Source: CAD feature listing. Evaluate the final solid. Frame: model axes, mm. A direction names the side the tool comes from. Round coordinates to 2 decimals unless told otherwise and drop trailing zeros.
```python
from build123d import *


with BuildPart() as part:
    # Sketch2 → Revolve2 (revolve)
    with BuildSketch(Plane(origin=(0, 0, 0), x_dir=(0, 0, -1), z_dir=(1, 0, 0)), mode=Mode.PRIVATE) as revolve2_sk:
        with BuildLine():
            Line((0, 0), (31, 0))
            Line((31, 0), (31, 9))
            Line((31, 9), (24.583151623, 9))
            ThreePointArc((24.583151623, 9), (19.839895343, 11.325558565), (18.773545819, 16.499493381))
            Line((18.773545819, 16.499493381), (22, 29))
            Line((22, 29), (22, 35))
            Line((22, 35), (18, 35))
            Line((18, 35), (13.354094276, 17))
            Line((13.354094276, 17), (8.876757203, 17))
            Line((8.876757203, 17), (4, 34.552318614))
            Line((4, 34.552318614), (0, 34.552318614))
            Line((0, 34.552318614), (0, 28.552318614))
            Line((0, 28.552318614), (4.37578125, 12.803101771))
            ThreePointArc((4.37578125, 12.803101771), (3.873716269, 10.184690841), (1.485274798, 9))
            Line((1.485274798, 9), (0, 9))
            Line((0, 9), (0, 0))
        make_face()
    revolve(revolve2_sk.sketch.rotate(Axis((0, -15, 0), (0, 0, -1)), 90), axis=Axis((0, -15, 0), (0, 0, -1)))


solid = part.part
```
Q1. Line query: line 1 (Y direction, x = 0, z = -10); line 2 (Y direction, x = 0, z = -18.5); line 3 (Z direction, x = -46, y = -22). Output: solid intervals per line, ascending.
Q2. Set-up query: faces 1 (the face through (22.89, -22.21, -27.75)), 2 (the face through (47.264, -29.884, -1.972)), 3 (the face through (-4.28, -47.59, -13.58)). Return all of +Z, -Z, +X, -X, +Y, -Y with unobstructed straight access to the full face (end or side cutting, diameter ignored); none if empty.
Q3. Pin query (flat end, axial travel): P1, Ø2, axis at x = -21, z = -12, coming from the +Y side; P2, Ø1, axis at x = -29, y = -10, coming from the -Z side; P3, Ø3, axis at y = 2.5, z = -21, coming from the +X side. Return the tip coordinate at first contact, or that it passes through.
Q4. Mould query, pull axis Z, two halves, no side actions, for faces 4 (the face through (-6.94, 16.24, -11.08)), 5 (the face through (0.2, 29.2, -22)), 6 (the face through (31.57, -24.94, -8.57)), 7 (the face through (47.69, -30.02, -19.97)). Classes: pulls with the +Z half, pulls with the -Z half, needs draft (parallel to the pull), parting line crosses it, or undercut.
Filled in:
1. line 1: y = -47 to -30, 0 to 17
1. line 2: y = -65 to -30, 0 to 35
1. line 3: z = -22 to -17.1, -4.84 to 0
2. face 1: -Z
2. face 2: +Z
2. face 3: none
3. P1: stops at y = 9.98
3. P2: stops at z = -18.68
3. P3: stops at x = 47.37
4. face 4: undercut
4. face 5: pulls with the -Z half
4. face 6: undercut
4. face 7: needs draft
